Autodesk Inventor part; units mm, degrees
ref_plane "YZ Plane" through (0, 0, 0) normal (1, 0, 0) x (0, 1, 0)
ref_plane "XZ Plane" through (0, 0, 0) normal (0, 1, 0) x (-1, 0, 0)
ref_plane "XY Plane" through (0, 0, 0) normal (0, 0, 1) x (1, 0, 0)
sketch "Sketch1" plane through (0, 0, 0) normal (1, 0, 0) x (0, 1, 0)
  line L0 (-25.4, -65.0875) -> (25.4, -65.0875)
  line L1 (25.4, -65.0875) -> (25.4, 65.0875)
  line L2 (25.4, 65.0875) -> (-25.4, 65.0875)
  line L3 (-25.4, 65.0875) -> (-25.4, -65.0875)
  line L4 (-25.4, -65.0875) -> (25.4, 65.0875) construction
  line L5 (25.4, -65.0875) -> (-25.4, 65.0875) construction
  point P0 (0, 0)
  dimension "d0" = 130.175
  dimension "d1" = 50.8
extrude "Extrusion1" add sketch "Sketch1" along normal blind 6.35
sketch "Sketch2" plane through (6.35, 0, 0) normal (1, 0, 0) x (0, 0, -1)
  line L0 (-50.8, 17.4625) -> (-50.8, -17.4625) construction
  line L1 (-65.0875, 25.4) -> (-65.0875, -25.4) construction
  line L2 (65.0875, 25.4) -> (65.0875, -25.4) construction
  line L3 (65.0875, -25.4) -> (-65.0875, -25.4) construction
  line L4 (-65.0875, 25.4) -> (65.0875, 25.4) construction
  line L5 (-65.0875, -25.4) -> (-65.0875, 25.4)
  point P0 (0, 0)
  point P1 (-38.1, 0)
  point P2 (-50.8, 0)
  point P3 (-65.0875, 0)
  point P4 (-25.4, 17.4625)
  point P5 (-12.7, 0)
  point P6 (-25.4, -17.4625)
  point P7 (0, 17.4625)
  point P8 (12.7, 0)
  point P9 (0, -17.4625)
  point P10 (25.4, 17.4625)
  point P11 (38.1, 0)
  point P12 (25.4, -17.4625)
  point P13 (50.8, 17.4625)
  point P14 (63.5, 0)
  point P15 (50.8, -17.4625)
  dimension "d6" = 34.925
  dimension "d7" = 14.2875
  dimension "d8" = 12.7
  dimension "d11" = 25.4
hole "Hole1" at (6.35, -17.4625, 50.8) at (6.35, 17.4625, 50.8) at (6.35, 0, 38.1) at (6.35, 17.4625, 25.4) at (6.35, 0, 12.7) at (6.35, -17.4625, 25.4) at (6.35, 17.4625, 0) at (6.35, 0, -12.7) at (6.35, -17.4625, 0) at (6.35, 17.4625, -25.4) at (6.35, -17.4625, -25.4) at (6.35, 0, -38.1) at (6.35, 17.4625, -50.8) at (6.35, -17.4625, -50.8) direction (-1, 0, 0) diameter 4.3434 end through all
fillet "Fillet1" radius 3.175 4 edges at (3.175, 25.4, 65.0875) (3.175, 25.4, -65.0875) (3.175, -25.4, -65.0875) (3.175, -25.4, 65.0875)
properties part number "CL4-021" material "Aluminum 6061"
The model under review builds one solid part; all positions refer to its coordinate system, in mm. Round coordinates to 2 decimals unless told otherwise and drop trailing zeros. Loops run counter-clockwise (first coordinate to the right, second up) from the corner with the lowest first, then second, coordinate; pieces in that order, holes last. Notation, with made-up numbers: (-24, 22) -> (11, 22) arc R19 ccw to (11, 27) -> close; hole circle Ø10 at (6, 55). An arc over 180 degrees is marked (long way). Answer in a Markdown table with one row per item.
1) For pin 1 Ø4 at (y, z) = (17.46, -25.4) entering from -X, flat-tipped, find the tip position at first contact; note if it passes through.
Taken from the geometry:
| item | result |
|---|---|
| pin 1 | passes through |
2) Draft analysis for pull direction Z (two halves, no side actions). For faces 1 (the flat face through (0, 0, 1)), 2 (the cylindrical face through (3.22, -24.45, 64.18)), 3 (the cylindrical face through (3.131, -16.631, 23.394)), state which applies: pulls with the +Z half, pulls with the -Z half, needs draft (parallel to the pull), parting line crosses it, or undercut.
Taken from the geometry:
| item | result |
|---|---|
| face 1 | needs draft |
| face 2 | pulls with the +Z half |
| face 3 | undercut |
3) Consider section C-C, the plane y = 0. Write out the cut boundary in (x, z).
Taken from the geometry:
| item | result |
|---|---|
| outline | (0, -65.09) -> (6.35, -65.09) -> (6.35, -40.27) -> (0, -40.27) -> close; (0, -35.93) -> (6.35, -35.93) -> (6.35, -14.87) -> (0, -14.87) -> close; (0, -10.53) -> (6.35, -10.53) -> (6.35, 10.53) -> (0, 10.53) -> close; (0, 14.87) -> (6.35, 14.87) -> (6.35, 35.93) -> (0, 35.93) -> close; (0, 40.27) -> (6.35, 40.27) -> (6.35, 65.09) -> (0, 65.09) -> close |
4) Wall thickness on line 1 along Z through (x, y) = (4.5, 0); line 2 along Z through (x, y) = (3.25, -19); line 3 along Y through (x, z) = (2.25, -50.8): over which ranges is each line inside the solid? List them lowest first.
Taken from the geometry:
| item | result |
|---|---|
| line 1 | z = -65.09 to -40.27, -35.93 to -14.87, -10.53 to 10.53, 14.87 to 35.93, 40.27 to 65.09 |
| line 2 | z = -65.09 to -52.33, -49.27 to -26.93, -23.87 to -1.53, 1.53 to 23.87, 26.93 to 49.27, 52.33 to 65.09 |
| line 3 | y = -25.4 to -19.63, -15.29 to 15.29, 19.63 to 25.4 |
5) Consider section A-A, the plane z = 50.8. Write out the cut boundary in (x, y).
Taken from the geometry:
| item | result |
|---|---|
| outline | (0, -25.4) -> (6.35, -25.4) -> (6.35, -19.63) -> (0, -19.63) -> close; (0, -15.29) -> (6.35, -15.29) -> (6.35, 15.29) -> (0, 15.29) -> close; (0, 19.63) -> (6.35, 19.63) -> (6.35, 25.4) -> (0, 25.4) -> close |
6) Consider section D-D, the plane x = 2.75. Count the separate pieces of the cut face and the enclosed holes in it, plus the area to 3 significant figures.
Taken from the geometry:
| item | result |
|---|---|
| separate pieces | 1 |
| enclosed holes | 14 |
| area | 6,400 mm² |
7) Consider section B-B, the plane z = -12.7. Write out the cut boundary in (x, y), plus the area to 3 significant figures.
Taken from the geometry:
| item | result |
|---|---|
| outline | (0, -25.4) -> (6.35, -25.4) -> (6.35, -2.17) -> (0, -2.17) -> close; (0, 2.17) -> (6.35, 2.17) -> (6.35, 25.4) -> (0, 25.4) -> close |
| area | 295 mm² |
